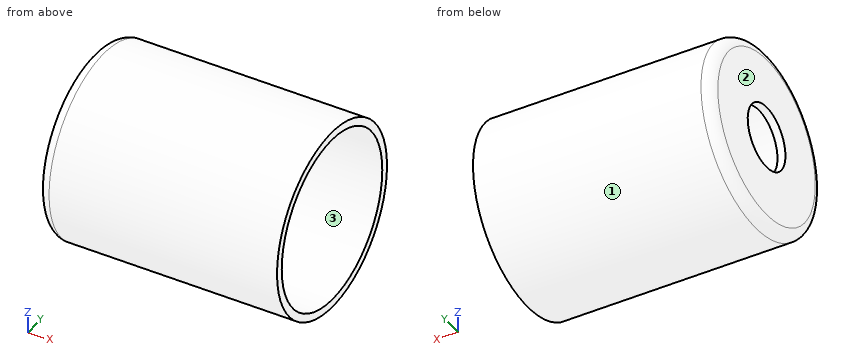
Autodesk Inventor part; units mm, degrees
ref_plane "YZ Plane" through (0, 0, 0) normal (1, 0, 0) x (0, 1, 0)
ref_plane "XZ Plane" through (0, 0, 0) normal (0, 1, 0) x (-1, 0, 0)
ref_plane "XY Plane" through (0, 0, 0) normal (0, 0, 1) x (1, 0, 0)
sketch "Sketch1" plane through (0, 0, 0) normal (1, 0, 0) x (0, 1, 0)
  circle A0 centre (0, 0) radius 17.5
  dimension "d0" = 35
extrude "Extrusion1" add sketch "Sketch1" along normal blind 45
shell "Shell1" thickness 1.5 removed faces 1 at (45, 4.865, -5.1831)
sketch "Sketch2" plane through (0, 0, 0) normal (-1, 0, 0) x (0, 0, 1)
  point P0 (0, 0)
hole "Hole1" at (0, 0, 0) direction (1, 0, 0) diameter 12 end through all
fillet "Fillet1" radius 2 2 edges at (0, -17.5, 0) (1.5, -16, 0)
properties material "Steel, Mild"
Geometry: final body of the model. Coordinates: model frame, mm. Face numbers are marked on the shaded views. Coordinates: 2 decimals unless noted, no trailing zeros. Order: outer loops, then holes, each group sorted by start corner. A loop starts at its lowest first (then second) coordinate and runs counter-clockwise, first axis right, second up. Notation, with made-up numbers: (83.5, 13) -> (121.5, 13) arc R14 ccw to (121.5, 32) -> close; hole circle Ø3 at (25, 39.25). An arc over 180 degrees is marked (long way). Write each question's results on one line, items separated by ' | '. Start each with the question number.
1) Material intervals for line 1 along Z through (x, y) = (32, 0); line 2 along Y through (x, z) = (28.5, 0.5); line 3 along X through (y, z) = (-2, 8), sorted ascending.
2) Cut plane C-C, the plane x = 17.5. Output: boundary loops of the cut face in (y, z), and give its area (3 significant figures).
3) First-contact query: pin 1 (1.5 mm diameter, centred on x = 37.5, z = -4.5, fed in from +Y); pin 2 (6 mm diameter, centred on y = 0, z = 6, fed in from +X); pin 3 (5 mm diameter, centred on x = 40, z = -10.5, fed in from -Y). Flat tips, straight axial feed; report the tip coordinate or a pass-through.
4) Cut plane A-A, the plane z = 0. Output: boundary loops of the cut face in (x, y), and give its area (3 significant figures).
5) Mould query, pull axis Z, two halves, no side actions, for the marked faces 1, 2 and 3. Classes: released by +Z, released by -Z, zero draft, split by the parting line, or undercut.
Checks:
1) line 1: -17.5 to -16, 16 to 17.5 | line 2: -17.49 to -15.99, 15.99 to 17.49 | line 3: 0 to 1.5
2) outline: circle Ø35 at (0, 0); hole circle Ø32 at (0, 0) | area: 158 mm^2
3) pin 1: y = 17.09 | pin 2: x = 1.5 | pin 3: y = -15.56
4) outline: (0, -15.5) arc R2 ccw to (2, -17.5) -> (45, -17.5) -> (45, -16) -> (3.5, -16) arc R2 cw to (1.5, -14) -> (1.5, -6) -> (0, -6) -> close; (0, 6) -> (1.5, 6) -> (1.5, 14) arc R2 cw to (3.5, 16) -> (45, 16) -> (45, 17.5) -> (2, 17.5) arc R2 ccw to (0, 15.5) -> close | area: 165 mm^2
5) face 1: split by the parting line | face 2: zero draft | face 3: undercut
